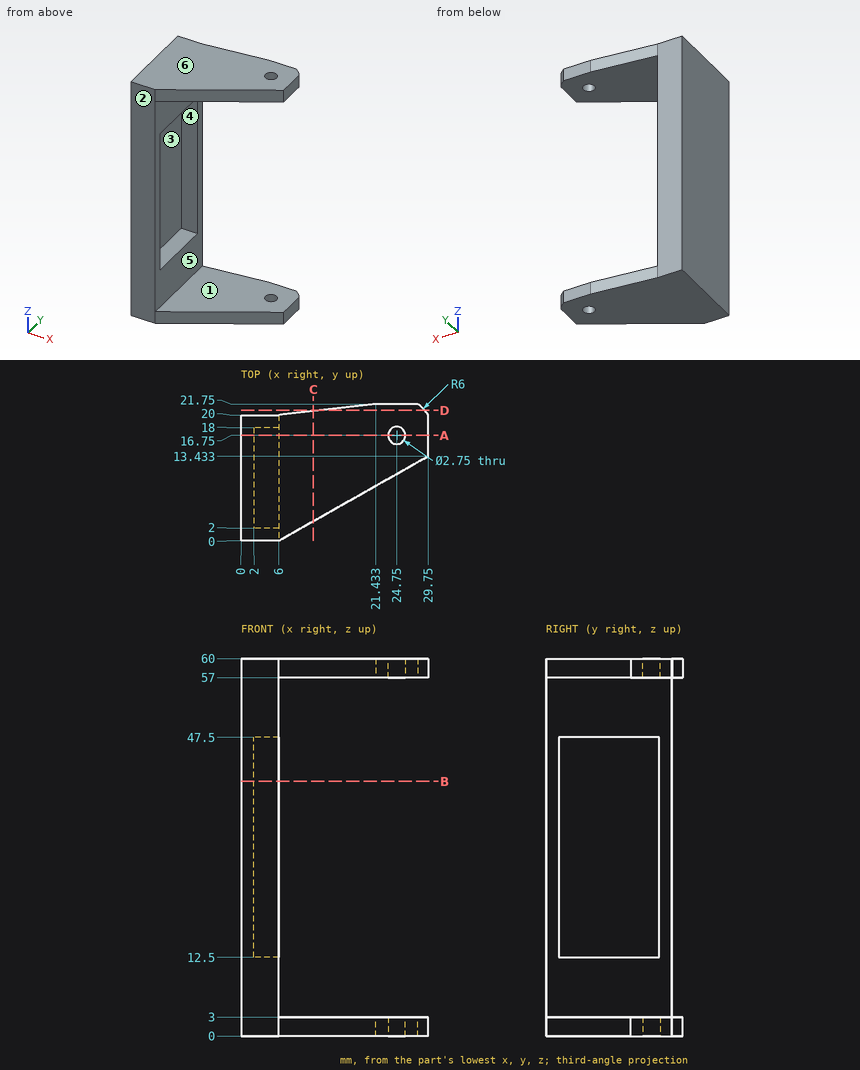
Drawing for the job (mm, zero at the part's lowest x, y, z). A direction names the side the tool comes from. Round coordinates to 2 decimals unless told otherwise and drop trailing zeros. Loops run counter-clockwise (first coordinate to the right, second up) from the corner with the lowest first, then second, coordinate; pieces in that order, holes last. Notation, with made-up numbers: (79, -12) - (129, -12) arc R13 ccw to (129, -3) - close; hole circle Ø5 at (29.25, 73.25). An arc over 180 degrees is marked (long way). Write each question's results on one line, items separated by ' | '.
(1) Saw through at D-D, the plane y = 20.75. List the corners of the cut face in (x, z) (1 decimal).
Answer below:
outline: (12.6, 0) - (29.2, 0) - (29.2, 3) - (12.6, 3) - close; (12.6, 57) - (29.2, 57) - (29.2, 60) - (12.6, 60) - close
(2) Saw through at A-A, the plane y = 16.75. Count the separate pieces of the cut face and the enclosed holes in it, then the cut area to 3 significant figures.
Answer below:
separate pieces: 3 | enclosed holes: 0 | area: 346 mm^2
(3) Saw through at C-C, the plane x = 11.5. List the corners of the cut face in (y, z).
Answer below:
outline: (3.11, 0) - (20.62, 0) - (20.62, 3) - (3.11, 3) - close; (3.11, 57) - (20.62, 57) - (20.62, 60) - (3.11, 60) - close
(4) Pin check, flat tips, straight feed: pin 1 (10 mm diameter, centred on y = 12, z = 11, fed in from -X); pin 2 (1.5 mm diameter, centred on y = 13, z = 16, fed in from +X); pin 3 (10 mm diameter, centred on y = 18.5, z = 28.5, fed in from +X); pin 4 (6.5 mm diameter, centred on x = 3, z = 42, fed in from +Y). Stop position of each tip, or through.
Answer below:
pin 1: stops at x = 0 | pin 2: stops at x = 2 | pin 3: stops at x = 6 | pin 4: stops at y = 20
(5) Saw through at B-B, the plane z = 40.5. List the corners of the cut face in (x, y).
Answer below:
outline: (0, 0) - (6, 0) - (6, 2) - (2, 2) - (2, 18) - (6, 18) - (6, 20) - (0, 20) - close
(6) Mould opens along Y. For the marked faces 1, 2 and 3 say: released by +Y, released by -Y, zero draft, split by the parting line, or undercut.
Answer below:
face 1: zero draft | face 2: released by -Y | face 3: undercut
(7) Wall check: L1, parallel to Z at x = 19, y = 16; L2, parallel to Z at x = 2.5, y = 11; L3, parallel to Y at x = 4.5, z = 42.5. Give the ranges that are in metal, low to high.
Answer below:
L1: z = 0 to 3, 57 to 60 | L2: z = 0 to 12.5, 47.5 to 60 | L3: y = 0 to 2, 18 to 20
(8) 3-axis set-ups, long thin cutter, end or side, ignore diameter. For the marked faces 4, 5 and 6: which of +Z, -Z, +X, -X, +Y, -Y reach the whole face in a straight line?
Answer below:
face 4: +X | face 5: +X, +Y, -Y | face 6: +Z, +X, -X, +Y, -Y
